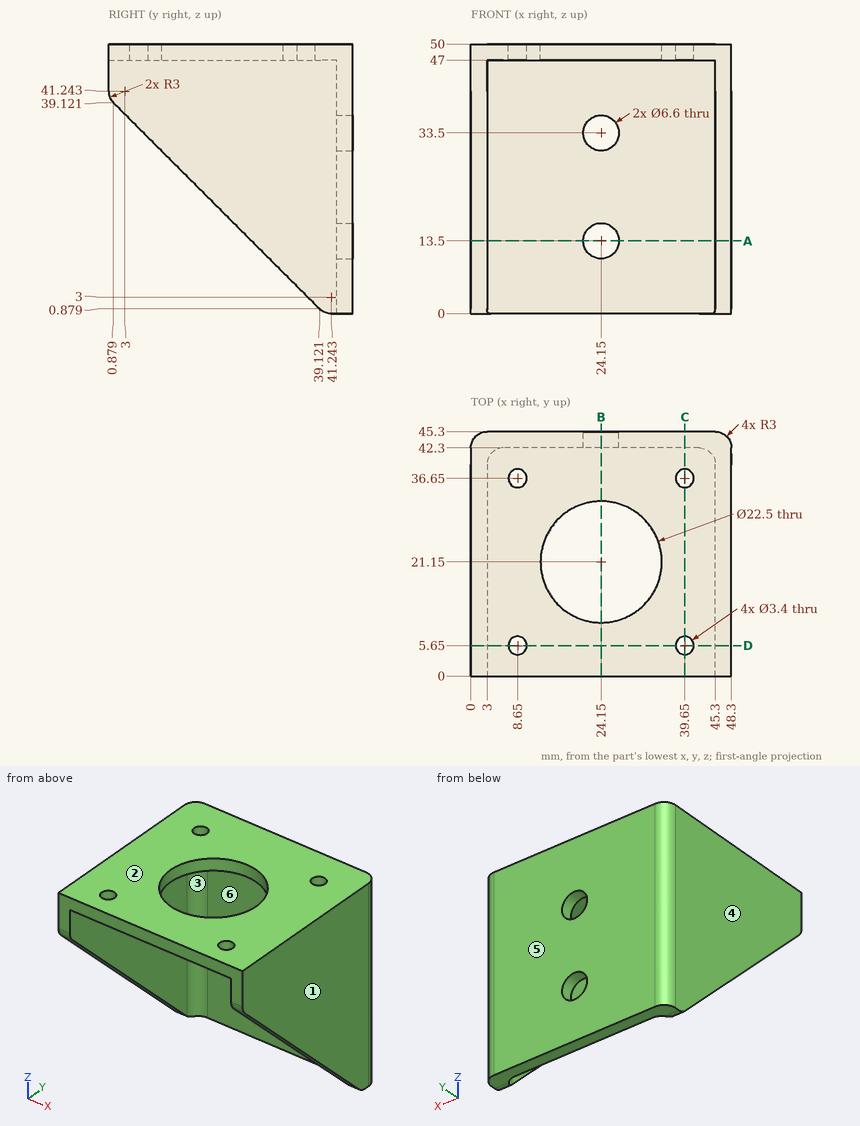
Design review of the part shown in the three views and the two pictorial views. Dimensions are in mm from the part's minimum x, y and z. A direction names the side the tool comes from. Round coordinates to 2 decimals unless told otherwise and drop trailing zeros. Write each loop counter-clockwise with the first axis right and the second up, starting at its lowest first coordinate (ties: lowest second). Pieces come first, ordered by that corner, then holes. Notation, with made-up numbers: M 60,-34 L 109,-34 A25 ccw 109,-3 Z; hole C 22,-1.75 d5. An arc over 180 degrees is marked long. One line per item, written item: value. Start each with the question number.
1. For the marked faces 5 and 6, list the 3-axis set-ups (+Z, -Z, +X, -X, +Y, -Y) from which the entire face can be reached by the end or side of a thin tool; tool diameter is ignored.
2. Take a section at C-C on x = 39.65. State the section outline as (y, z) points.
3. To check wall thickness, follow probe 1 along X at (y, z) = (36.65, 48.6); probe 2 along Y at (x, z) = (39.65, 48.1); probe 3 along Z at (x, y) = (24.15, 44.25). State the ranges of each line that lie inside material, in increasing order. Write a range as from..to.
4. Take a section at A-A on z = 13.5. State the section outline as (x, y) points.
5. Take a section at B-B on x = 24.15. State the section outline as (y, z) points, then the cut area to 3 significant figures.
6. Draft analysis for pull direction X (two halves, no side actions). For the marked faces 1, 2, 3 and 4, state which applies: pulls with the +X half, pulls with the -X half, needs draft (parallel to the pull), parting line crosses it, or undercut.
7. Clearance check with flat-ended pins moving along their axes: P1, Ø12, axis at x = 16.5, z = 14.5, coming from the -Y side; P2, Ø6, axis at x = 32, y = 26, coming from the -Z side; P3, Ø4, axis at x = 8.65, y = 5.65, coming from the +Z side; P4, Ø13.5, axis at x = 24.15, y = 21.15, coming from the -Z side. State where each tip first meets the part, or that it passes through.
8. Take a section at D-D on y = 5.65. State the section outline as (x, z) points.
Computed:
1. face 5: +Z, -Z, +X, -X, +Y
1. face 6: -Z, -Y
2. outline: M 0,47 L 3.95,47 L 3.95,50 L 0,50 Z; M 7.35,47 L 34.95,47 L 34.95,50 L 7.35,50 Z; M 38.35,47 L 42.3,47 L 42.3,0 L 45.3,0 L 45.3,50 L 38.35,50 Z
3. probe 1: x = 0..6.95, 10.35..37.95, 41.35..48.3
3. probe 2: y = 0..3.95, 7.35..34.95, 38.35..45.3
3. probe 3: z = 0..10.2, 16.8..30.2, 36.8..50
4. outline: M 0,26.5 L 3,26.5 L 3,39.3 A3 cw 6,42.3 L 20.85,42.3 L 20.85,45.3 L 3,45.3 A3 ccw 0,42.3 Z; M 27.45,42.3 L 42.3,42.3 A3 cw 45.3,39.3 L 45.3,26.5 L 48.3,26.5 L 48.3,42.3 A3 ccw 45.3,45.3 L 27.45,45.3 Z
5. outline: M 0,47 L 9.9,47 L 9.9,50 L 0,50 Z; M 32.4,47 L 42.3,47 L 42.3,36.8 L 45.3,36.8 L 45.3,50 L 32.4,50 Z; M 42.3,0 L 45.3,0 L 45.3,10.2 L 42.3,10.2 Z; M 42.3,16.8 L 45.3,16.8 L 45.3,30.2 L 42.3,30.2 Z
5. area: 170 mm²
6. face 1: pulls with the +X half
6. face 2: needs draft
6. face 3: undercut
6. face 4: pulls with the -X half
7. P1: stops at y = 42.3
7. P2: stops at z = 47
7. P3: stops at z = 50
7. P4: passes through
8. outline: M 0,34.35 L 3,34.35 L 3,47 L 6.95,47 L 6.95,50 L 0,50 Z; M 10.35,47 L 37.95,47 L 37.95,50 L 10.35,50 Z; M 41.35,47 L 45.3,47 L 45.3,34.35 L 48.3,34.35 L 48.3,50 L 41.35,50 Z
